Geometry: see drawing. Coordinates: mm, zero at the bounding-box minimum. A direction names the side the tool comes from. Coordinates: 2 decimals unless noted, no trailing zeros. Loops run counter-clockwise (first coordinate to the right, second up) from the corner with the lowest first, then second, coordinate; pieces in that order, holes last. Notation, with made-up numbers: (-32, 82.25) -> (-11, 82.25) arc R9 ccw to (-11, 92.25) -> close; hole circle Ø11 at (-31, 82.25). An arc over 180 degrees is marked (long way). One line per question, with ' | ' between items. Start each with the question number.
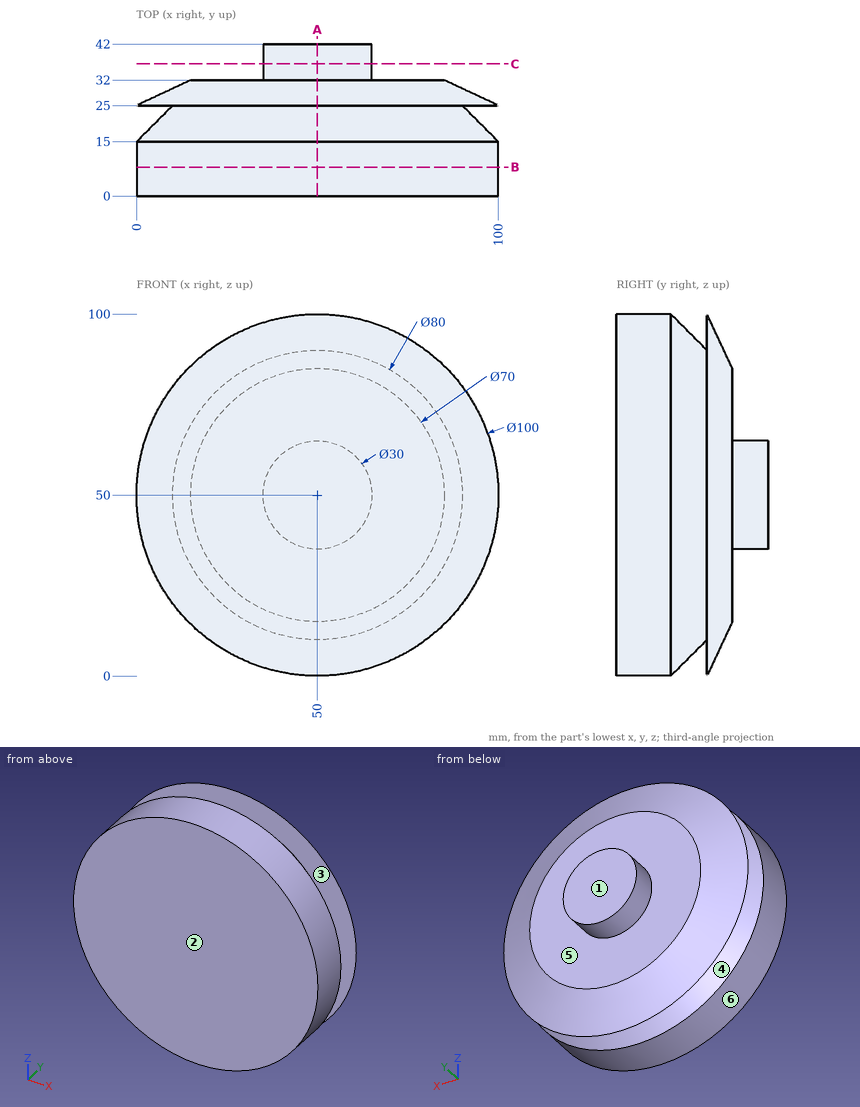
(1) Access query for the marked faces 4, 5 and 6. Directions: +Z, -Z, +X, -X, +Y, -Y. A direction counts if a zero-diameter tool reaches every point of the face in a straight line with its end or side. Return the directions, or none.
(2) Draft query along Y for the marked faces 1, 2 and 3. Return one class per face: pulls with the +Y half, pulls with the -Y half, needs draft (parallel to the pull), parting line crosses it, or undercut.
(3) Cut plane C-C, the plane y = 36.5. Return the cut outline in (x, z).
(4) Cut plane B-B, the plane y = 8. Return the cut outline in (x, z), and give its area (3 significant figures).
(5) Contact query for flat-ended pins moving along their axis: pin 1 Ø5 at (y, z) = (10.5, 80.5) entering from -X; pin 2 Ø3 at (x, z) = (39.5, 37) entering from +Y; pin 3 Ø4 at (y, z) = (34, 13.5) entering from +X; pin 4 Ø1.5 at (x, y) = (15, 21) entering from +Z. Output: stop coordinate, or through.
(6) Ray query, L1, parallel to Y at x = 61.5, z = 4; L2, parallel to Y at x = 25, z = 73; L3, parallel to Y at x = 22.5, z = 91. Return the intervals inside material, ascending.
(7) Cut plane A-A, the plane x = 50. Return the cut outline in (y, z), and give its area (4 significant figures).
Here are the results:
1) face 4: none | face 5: +Y | face 6: +Y, -Y
2) face 1: pulls with the +Y half | face 2: pulls with the -Y half | face 3: undercut
3) outline: circle Ø30 at (50, 50)
4) outline: circle Ø100 at (50, 50) | area: 7,850 mm2
5) pin 1: stops at x = 8.58 | pin 2: stops at y = 32 | pin 3: passes through | pin 4: stops at z = 78.2
6) L1: y = 0 to 17.58, 25 to 26.21 | L2: y = 0 to 32 | L3: y = 0 to 15.63, 25 to 25.29
7) outline: (0, 0) -> (15, 0) -> (25, 10) -> (25, 0) -> (32, 15) -> (32, 35) -> (42, 35) -> (42, 65) -> (32, 65) -> (32, 85) -> (25, 100) -> (25, 90) -> (15, 100) -> (0, 100) -> close | area: 3,295 mm2
